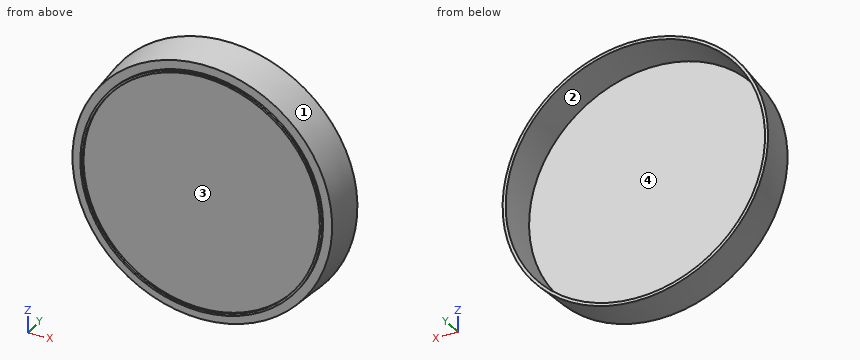
from build123d import *

# Parameters (mm, degrees)
SHELL1_T            = -1.016
SKETCH3_R           = 40.8305
SKETCH3_R_2         = 40.1447
BOSS_EXTRUDE1_DEPTH = 0.762


with BuildPart() as part:
    # Sketch2 → Revolve1 (revolve)
    with BuildSketch(Plane.XY, mode=Mode.PRIVATE) as revolve1_sk:
        Polygon((0, 0), (43.8785, 0), (44.8564, 14.1224), (0, 14.1224), align=None)
    revolve(revolve1_sk.sketch.rotate(Axis((0, 0, 0), (0, 1, 0)), 90), axis=Axis((0, 0, 0), (0, 1, 0)))

    # Shell1
    shell1_openings = [part.faces().sort_by_distance(p)[0] for p in [
        (0, 14.1224, 0),
    ]]
    offset(amount=SHELL1_T, openings=shell1_openings, kind=Kind.INTERSECTION)

    # Sketch3 → Boss-Extrude1 (add)
    with BuildSketch(Plane.XZ):
        with Locations(Location((0, 0, 0), (0, 0, 90))):
            Circle(SKETCH3_R)
        with Locations(Location((0, 0, 0), (0, 0, 90))):
            Circle(SKETCH3_R_2, mode=Mode.SUBTRACT)
    extrude(amount=BOSS_EXTRUDE1_DEPTH)


solid = part.part
Design review of the part built by this model. Coordinates are the model's own, in mm. Face numbers are marked on the shaded views. A direction names the side the tool comes from. Give positions to 0.01 mm unless a question says otherwise; leave off trailing zeros. Order: outer loops, then holes, each group sorted by start corner. A loop starts at its lowest first (then second) coordinate and runs counter-clockwise, first axis right, second up. Notation, with made-up numbers: (46.5, 37.5) - (92.5, 37.5) arc R14 ccw to (92.5, 44.5) - close; hole circle Ø2 at (-11.75, 50). An arc over 180 degrees is marked (long way). Use CSV: the item, a comma, the result in double quotes. Start each with the question number.
Q1. Machinability: for the marked faces 3 and 4, which of the approach directions +Z, -Z, +X, -X, +Y, -Y give a long, thin tool a straight path to every point of the face, cutting with its end or side? Answer none if there is none.
Q2. Take a section at B-B (x = 0). State the section outline as (y, z) points, and give its area (3 significant figures).
Q3. Take a section at A-A (z = 0). State the section outline as (x, y) points, and give its area (3 significant figures).
Q4. For line 1 (X direction, y = -0.5, z = 0); line 2 (Y direction, x = 4, z = 31.5); line 3 (Y direction, x = -17, z = -36.5), list the stretches that pass through material, from the lowest coordinate up.
Q5. Draft analysis for pull direction X (two halves, no side actions). For the marked faces 1 and 2, state which applies: pulls with the +X half, pulls with the -X half, needs draft (parallel to the pull), parting line crosses it, or undercut.
Q6. For P1, Ø8, axis at y = 5.5, z = -19.5, coming from the +X side; P2, Ø2, axis at y = 5.5, z = 13.5, coming from the -X side; P3, Ø3, axis at x = 3.5, z = 0.5, coming from the -Y side, all flat-tipped, find the tip position at first contact; note any pin that passes through.
Calculated:
1,face 3,"-Y"
1,face 4,"+Y"
2,outline,"(-0.76, -40.83) - (0, -40.83) - (0, -43.88) - (14.12, -44.86) - (14.12, -43.84) - (1.02, -42.93) - (1.02, 42.93) - (14.12, 43.84) - (14.12, 44.86) - (0, 43.88) - (0, 40.83) - (-0.76, 40.83) - (-0.76, 40.14) - (0, 40.14) - (0, -40.14) - (-0.76, -40.14) - close"
2,area,"117 mm²"
3,outline,"(-44.86, 14.12) - (-43.88, 0) - (-40.83, 0) - (-40.83, -0.76) - (-40.14, -0.76) - (-40.14, 0) - (40.14, 0) - (40.14, -0.76) - (40.83, -0.76) - (40.83, 0) - (43.88, 0) - (44.86, 14.12) - (43.84, 14.12) - (42.93, 1.02) - (-42.93, 1.02) - (-43.84, 14.12) - close"
3,area,"117 mm²"
4,line 1,"x = -40.83 to -40.14, 40.14 to 40.83"
4,line 2,"y = 0 to 1.02"
4,line 3,"y = -0.76 to 1.02"
5,face 1,"parting line crosses it"
5,face 2,"undercut"
6,P1,"stops at x = 41.49"
6,P2,"stops at x = -42.47"
6,P3,"stops at y = 0"
